Verification items for the finished model (mm, model axes). Face numbers are marked on the shaded views. A direction names the side the tool comes from. Give positions to 0.01 mm unless a question says otherwise; leave off trailing zeros. Order: outer loops, then holes, each group sorted by start corner. A loop starts at its lowest first (then second) coordinate and runs counter-clockwise, first axis right, second up.
(1) Mould release check, pull along X, two halves, no side actions. Record for the marked faces 4, 5, 6 and 7: pulls with the +X half, pulls with the -X half, needs draft (parallel to the pull), parting line crosses it, or undercut.
(2) Scan lines: L1, parallel to Y at x = 57, z = 6.25; L2, parallel to X at y = 29.5, z = 5.5; L3, parallel to Y at x = 50.5, z = 5.75. Record each from-to range of solid material in increasing order.
(3) Sectioned sample at B-B on z = 2.75. Record the cut outline in (x, y) (3 decimals), plus the area to 3 significant figures.
(4) Access from +Z, -Z, +X, -X, +Y, -Y to the whole of each face (thin tool, end or side, straight path). Record for the marked faces 1, 2 and 3.
(5) Sectioned sample at D-D on z = 11.25. Record the cut outline in (x, y), plus the area to 3 significant figures.
(6) Sectioned sample at A-A on y = 23. Record the cut outline in (x, z) (3 decimals).
(7) Gauge pin test, flat ends, axial feed: pin 1 (4.5 mm diameter, centred on x = 31, z = 24.5, fed in from -Y); pin 2 (1.5 mm diameter, centred on x = 69.5, y = 23.5, fed in from +Z); pin 3 (2 mm diameter, centred on x = 39.5, z = 23.5, fed in from +Y). Record the tip position at first contact, or that the pin passes through.
(8) Sectioned sample at C-C on y = 8. Record the cut outline in (x, z) (3 decimals), plus the area to 3 significant figures.
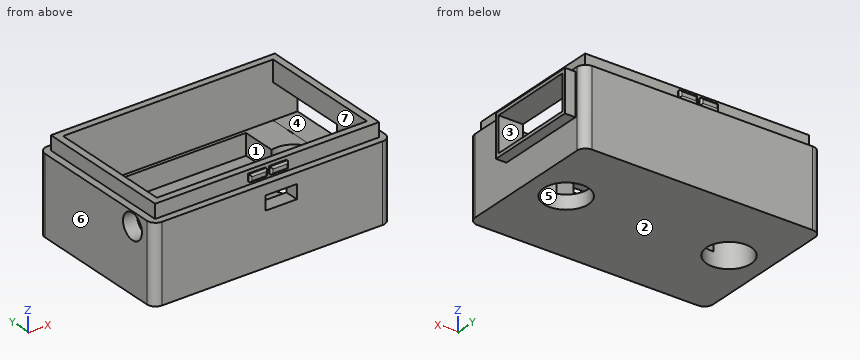
```python
from build123d import *

# Parameters (mm, degrees)
SKETCH1_W                   = 68
SKETCH1_H                   = 44
MIAN_BOSS_EXTRUDE_DEPTH     = 26
SKETCH2_W                   = 60
SKETCH2_H                   = 36
MAIN_CUT_DEPTH              = 16
SKETCH4_W                   = 45
SKETCH4_H                   = 35
BATTERY_CUT_DEPTH           = 6
SKETCH5_R                   = 6.375
ELCTRODE_CUT_DEPTH          = 12
SKETCH6_W                   = 9.989337028
SKETCH6_H                   = 24.5
USB_C_CUT_DEPTH             = 7
SKETCH7_R                   = 3.625
BUTTON_CUT_DEPTH            = 7
SKETCH8_W                   = 9
SKETCH8_H                   = 4
SWITCH_CUT_DEPTH            = 7
OUTSIDE_FILLET_R            = 2.5
SKETCH10_OUTSIDE_W          = 87.012
SKETCH10_OUTSIDE_H          = 63.012
SKETCH10_OUTSIDE_W_2        = 64
SKETCH10_OUTSIDE_H_2        = 40
OUTER_LID_EXTRUDE_DEPTH     = 4
LID_SNAP_EXTRUDE_DEPTH      = 1
LID_SNAP_EXTRUDE_DEPTH_BACK = 41
SKETCH11_W                  = 5
SKETCH11_H                  = 2
SKETCH13_W                  = 11
SKETCH13_H                  = 36
INNER_LID_EXTRUDE_DEPTH     = 3
SKETCH14_W                  = 11.989337028
SKETCH14_H                  = 26.5
SKETCH14_W_2                = 9.989337028
SKETCH14_H_2                = 24.5
USB_COVER_EXTRUDE_DEPTH     = 3
LID_SNAP_FILLET_R           = 0.5


with BuildPart() as part:
    # Sketch1 → Mian Boss Extrude (new body)
    with BuildSketch(Plane.XY):
        with Locations((34, 22)):
            Rectangle(SKETCH1_W, SKETCH1_H)
    extrude(amount=MIAN_BOSS_EXTRUDE_DEPTH)

    # Sketch2 → Main cut (cut)
    with BuildSketch(Plane.XY.offset(26)):
        with Locations((34, 22)):
            Rectangle(SKETCH2_W, SKETCH2_H)
    extrude(amount=-MAIN_CUT_DEPTH, mode=Mode.SUBTRACT)

    # Sketch4 → Battery Cut (cut)
    with BuildSketch(Plane.XY.offset(10)):
        with Locations((33, 21.5)):
            Rectangle(SKETCH4_W, SKETCH4_H)
    extrude(amount=-BATTERY_CUT_DEPTH, mode=Mode.SUBTRACT)

    # Sketch5 → Elctrode Cut (cut)
    with BuildSketch(Plane(origin=(0, 0, 0), x_dir=(-1, 0, 0), z_dir=(0, 0, -1))):
        with Locations((-57.25, 23)):
            Circle(SKETCH5_R)
        with Locations((-10.75, 23)):
            Circle(SKETCH5_R)
    extrude(amount=-ELCTRODE_CUT_DEPTH, mode=Mode.SUBTRACT)

    # Sketch6 → USB-c Cut (cut)
    with BuildSketch(Plane(origin=(68, 0, 0), x_dir=(0, 0, -1), z_dir=(1, 0, 0))):
        with Locations((-15.005331486, 27.75)):
            Rectangle(SKETCH6_W, SKETCH6_H)
    extrude(amount=-USB_C_CUT_DEPTH, mode=Mode.SUBTRACT)

    # Sketch7 → Button Cut (cut)
    with BuildSketch(Plane.ZY):
        with Locations((18, 8)):
            Circle(SKETCH7_R)
    extrude(amount=-BUTTON_CUT_DEPTH, mode=Mode.SUBTRACT)

    # Sketch8 → Switch Cut (cut)
    with BuildSketch(Plane.XZ):
        with Locations((36.5, 17)):
            Rectangle(SKETCH8_W, SKETCH8_H)
    extrude(amount=-SWITCH_CUT_DEPTH, mode=Mode.SUBTRACT)

    # Outside Fillet
    outside_fillet_edges = [part.edges().sort_by_distance(p)[0] for p in [
        (0, 44, 13),
        (68, 44, 13),
        (68, 0, 13),
        (0, 0, 13),
    ]]
    fillet(outside_fillet_edges, radius=OUTSIDE_FILLET_R)

    # Sketch10 outside → Outer lid Extrude (cut)
    with BuildSketch(Plane.XY.offset(26)):
        with Locations((34, 22)):
            Rectangle(SKETCH10_OUTSIDE_W, SKETCH10_OUTSIDE_H)
        with Locations((34, 22)):
            Rectangle(SKETCH10_OUTSIDE_W_2, SKETCH10_OUTSIDE_H_2, mode=Mode.SUBTRACT)
    extrude(amount=-OUTER_LID_EXTRUDE_DEPTH, mode=Mode.SUBTRACT)

    # Sketch11 → Lid Snap-Extrude (add, two sides: drawn at the far end of the back side and taken through both)
    with BuildSketch(Plane.XZ.offset(-2).offset(-LID_SNAP_EXTRUDE_DEPTH_BACK)):
        with Locations((31, 24)):
            Rectangle(SKETCH11_W, SKETCH11_H)
        with Locations((37, 24)):
            Rectangle(SKETCH11_W, SKETCH11_H)
    extrude(amount=LID_SNAP_EXTRUDE_DEPTH + LID_SNAP_EXTRUDE_DEPTH_BACK)

    # Sketch13 → Inner Lid-Extrude (cut)
    with BuildSketch(Plane.XY.offset(25)):
        with Locations((34, 22)):
            Rectangle(SKETCH13_W, SKETCH13_H)
    extrude(amount=-INNER_LID_EXTRUDE_DEPTH, mode=Mode.SUBTRACT)

    # Sketch14 → USB Cover-Extrude (add)
    with BuildSketch(Plane(origin=(68, 0, 0), x_dir=(0, 0, -1), z_dir=(1, 0, 0))):
        with Locations((-15.005331486, 27.75)):
            Rectangle(SKETCH14_W, SKETCH14_H)
        with Locations((-15.005331486, 27.75)):
            Rectangle(SKETCH14_W_2, SKETCH14_H_2, mode=Mode.SUBTRACT)
    extrude(amount=USB_COVER_EXTRUDE_DEPTH)

    # Lid Snap Fillet
    lid_snap_fillet_edges = [part.edges().sort_by_distance(p)[0] for p in [
        (28.5, 43, 24),
        (31, 43, 25),
        (33.5, 43, 24),
        (31, 43, 23),
        (28.5, 1, 24),
        (31, 1, 23),
        (33.5, 1, 24),
        (31, 1, 25),
        (37, 43, 25),
        (39.5, 43, 24),
        (37, 43, 23),
        (34.5, 43, 24),
        (37, 1, 25),
        (34.5, 1, 24),
        (37, 1, 23),
        (39.5, 1, 24),
    ]]
    fillet(lid_snap_fillet_edges, radius=LID_SNAP_FILLET_R)


solid = part.part
```
Ans:
1. face 4: needs draft
1. face 5: undercut
1. face 6: pulls with the -X half
1. face 7: undercut
2. L1: y = 0 to 16.63, 29.37 to 44
2. L2: x = 0 to 10.5, 55.5 to 68
2. L3: y = 0 to 4, 39 to 44
3. outline: (0, 2.5) arc R2.5 ccw to (2.5, 0) - (65.5, 0) arc R2.5 ccw to (68, 2.5) - (68, 41.5) arc R2.5 ccw to (65.5, 44) - (2.5, 44) arc R2.5 ccw to (0, 41.5) - close; hole circle Ø12.75 at (10.75, 23); hole circle Ø12.75 at (57.25, 23)
3. area: 2,730 mm2
4. face 1: +Z
4. face 2: -Z, +X, -X, +Y, -Y
4. face 3: +X
5. outline: (0, 2.5) arc R2.5 ccw to (2.5, 0) - (65.5, 0) arc R2.5 ccw to (68, 2.5) - (68, 14.5) - (71, 14.5) - (71, 15.5) - (64, 15.5) - (64, 4) - (4, 4) - (4, 40) - (71, 40) - (71, 41) - (68, 41) - (68, 41.5) arc R2.5 ccw to (65.5, 44) - (2.5, 44) arc R2.5 ccw to (0, 41.5) - close
5. area: 735 mm2
6. outline: (0, 0) - (4.375, 0) - (4.375, 10) - (4, 10) - (4, 26) - (2, 26) - (2, 22) - (0, 22) - close; (17.125, 0) - (50.875, 0) - (50.875, 4) - (17.125, 4) - close; (63.625, 0) - (68, 0) - (68, 9.011) - (71, 9.011) - (71, 10.011) - (64, 10.011) - (64, 10) - (63.625, 10) - close; (64, 20) - (71, 20) - (71, 21) - (68, 21) - (68, 22) - (66, 22) - (66, 26) - (64, 26) - close
7. pin 1: stops at y = 1
7. pin 2: stops at z = 21
7. pin 3: stops at y = 43
8. outline: (0, 0) - (68, 0) - (68, 22) - (66, 22) - (66, 26) - (64, 26) - (64, 10) - (55.5, 10) - (55.5, 4) - (10.5, 4) - (10.5, 10) - (4, 10) - (4, 14.375) - (0, 14.375) - close; (0, 21.625) - (4, 21.625) - (4, 26) - (2, 26) - (2, 22) - (0, 22) - close
8. area: 493 mm2
